Build history of the part. All positions in model axes, mm. A direction names the side the tool comes from. Give positions to 0.01 mm unless a question says otherwise; leave off trailing zeros. Order: outer loops, then holes, each group sorted by start corner. A loop starts at its lowest first (then second) coordinate and runs counter-clockwise, first axis right, second up. Notation, with made-up numbers: (25, 74.25) - (32, 74.25) arc R9 cw to (32, 91.25) - close; hole circle Ø2 at (13, -33). An arc over 180 degrees is marked (long way). Write each question's results on one line, items separated by ' | '. Start each with the question number.
1) Cut at D-D on z = 3.55. List the corners of the cut face in (x, y), plus the area to 3 significant figures.
2) Tool access for faces 1 (the face through (-2.035, 34.598, 0.986)), 2 (the face through (11, 31.75, 4)), 3 (the face through (0, -8.6, 1.6)): list every direction of +Z, -Z, +X, -X, +Y, -Y with a clear straight run to the whole face (end or side of a thin tool).
3) Two-plate mould, pull along Y, no slides. Class faces 4 (the face through (-1.5, 0.07, 0.99)), 5 (the face through (6.79, -6.94, 3.97)), 6 (the face through (9.708, 16, 4)): +Y half, -Y half, draft (parallel to the pull), parting line (faces both ways), or undercut.
4) Cut at A-A on z = 0.8. List the corners of the cut face in (x, y).
5) Drill centre lines: line 1 along X through (y, z) = (18.5, 5.75); line 2 along Z through (x, y) = (3.5, 8); line 3 along Y through (x, z) = (2.5, 4.55). Where is each one in solid material? Low to high. Write a range as from..to.
6) Cut at C-C on y = 28. List the corners of the cut face in (x, z), plus the area to 3 significant figures.
7) Cut at B-B on y = -1. List the corners of the cut face in (x, z), plus the area to 3 significant figures.
8) Drop flat-ended pins along their axis: pin 1 Ø2 at (x, z) = (3, 5.5) entering from -Y; pin 2 Ø5 at (x, y) = (0, 0) entering from +Z; pin 3 Ø1.6 at (x, z) = (11, 4) entering from +Y. Give the stop position or say it passes through.
from build123d import *

# Parameters (mm, degrees)
SKETCH1_R           = 3.5
SKETCH1_R_2         = 1.5
BOSS_EXTRUDE1_DEPTH = 2
BOSS_EXTRUDE2_START = 2
BOSS_EXTRUDE2_DEPTH = 4


with BuildPart() as part:
    # Sketch1 → Boss-Extrude1 (new body)
    with BuildSketch(Plane.XY):
        with BuildLine():
            Line((9.70788, 31.75), (11.70788, 31.75))
            Line((11.70788, 31.75), (1.046303857, 35.089947341))
            ThreePointArc((1.046303857, 35.089947341), (2.820643854, 33.822189241), (3.5, 31.75))
            ThreePointArc((3.5, 31.75), (0, 28.25), (-3.5, 31.75))
            Line((-3.5, 31.75), (-3.5, 0))
            ThreePointArc((-3.5, 0), (0, 3.5), (3.5, 0))
            ThreePointArc((3.5, 0), (2.474873734, -2.474873734), (0, -3.5))
            Line((0, -3.5), (0, -9.70788))
            ThreePointArc((0, -9.70788), (6.864507779, -6.864507779), (9.70788, 0))
            Line((9.70788, 0), (9.70788, 31.75))
        make_face()
        with Locations((0, 31.75)):
            Circle(SKETCH1_R)
        with Locations((0, 31.75)):
            Circle(SKETCH1_R_2, mode=Mode.SUBTRACT)
        Circle(SKETCH1_R)
        Circle(SKETCH1_R_2, mode=Mode.SUBTRACT)
        with BuildLine():
            ThreePointArc((0, -9.70788), (6.864507779, -6.864507779), (9.70788, 0))
            Line((9.70788, 0), (9.70788, 31.75))
            Line((9.70788, 31.75), (11.70788, 31.75))
            Line((11.70788, 31.75), (11.70788, 0))
            ThreePointArc((11.70788, 0), (8.278721341, -8.278721341), (0, -11.70788))
            Line((0, -11.70788), (0, -9.70788))
        make_face()
    extrude(amount=BOSS_EXTRUDE1_DEPTH)

    # Sketch1<3> → Boss-Extrude2 (add)
    with BuildSketch(Plane.XY.offset(BOSS_EXTRUDE2_START)):
        with BuildLine():
            ThreePointArc((0, -9.70788), (6.864507779, -6.864507779), (9.70788, 0))
            Line((9.70788, 0), (9.70788, 31.75))
            Line((9.70788, 31.75), (11.70788, 31.75))
            Line((11.70788, 31.75), (11.70788, 0))
            ThreePointArc((11.70788, 0), (8.278721341, -8.278721341), (0, -11.70788))
            Line((0, -11.70788), (0, -9.70788))
        make_face()
    extrude(amount=BOSS_EXTRUDE2_DEPTH)


solid = part.part
Results:
1) outline: (0, -11.71) arc R11.71 ccw to (11.71, 0) - (11.71, 31.75) - (9.71, 31.75) - (9.71, 0) arc R9.71 cw to (0, -9.71) - close | area: 97.1 mm^2
2) face 1: +Z, -Z, +Y | face 2: +Z, +X, -X, +Y | face 3: +Z, -Z, -X, -Y
3) face 4: undercut | face 5: +Y half | face 6: draft
4) outline: (-3.5, 0) arc R3.5 ccw to (0, -3.5) - (0, -11.71) arc R11.71 ccw to (11.71, 0) - (11.71, 31.75) - (1.05, 35.09) arc R3.5 ccw to (-3.5, 31.75) - close; hole circle Ø3 at (0, 0); hole circle Ø3 at (0, 31.75)
5) line 1: 9.71..11.71 | line 2: 0..2 | line 3: -11.44..-9.38
6) outline: (-3.5, 0) - (11.71, 0) - (11.71, 6) - (9.71, 6) - (9.71, 2) - (-3.5, 2) - close | area: 38.4 mm^2
7) outline: (-3.35, 0) - (-1.12, 0) - (-1.12, 2) - (-3.35, 2) - close; (1.12, 0) - (11.67, 0) - (11.67, 6) - (9.66, 6) - (9.66, 2) - (1.12, 2) - close | area: 33.6 mm^2
8) pin 1: y = -11.54 | pin 2: z = 2 | pin 3: y = 31.75
